from build123d import *

# Parameters (mm, degrees)
ESBO_O1_W                = 20
ESBO_O1_H                = 3.5
RESSALTO_EXTRUS_O1_DEPTH = 22
ESBO_O2_W                = 18
ESBO_O2_H                = 3.80087929
CORTE_EXTRUS_O1_DEPTH    = 20.5
ESBO_O3_W                = 1
ESBO_O3_H                = 20.5
CORTE_EXTRUS_O2_DEPTH    = 1.5
ESBO_O4_W                = 20
ESBO_O4_H                = 1.5
RESSALTO_EXTRUS_O2_DEPTH = 10
ESBO_O5_R                = 1.5
CORTE_EXTRUS_O3_DEPTH    = 7
ESBO_O6_W                = 9
ESBO_O6_H                = 3.518504599
CORTE_EXTRUS_O4_DEPTH    = 2.5


with BuildPart() as part:
    # Esboço1 → Ressalto-extrusão1 (new body)
    with BuildSketch(Plane.XY):
        with Locations((17.16043247, -2.285464773)):
            Rectangle(ESBO_O1_W, ESBO_O1_H)
    extrude(amount=RESSALTO_EXTRUS_O1_DEPTH)

    # Esboço2 → Corte-extrusão1 (cut)
    with BuildSketch(Plane.XY.offset(22)):
        with Locations((17.16043247, -1.135025128)):
            Rectangle(ESBO_O2_W, ESBO_O2_H)
    extrude(amount=-CORTE_EXTRUS_O1_DEPTH, mode=Mode.SUBTRACT)

    # Esboço3 → Corte-extrusão2 (cut)
    with BuildSketch(Plane(origin=(0, -1.535464773, 0), x_dir=(1, 0, 0), z_dir=(0, 1, 0))):
        with Locations((7.66043247, -11.75)):
            Rectangle(ESBO_O3_W, ESBO_O3_H)
        with Locations((26.66043247, -11.75)):
            Rectangle(ESBO_O3_W, ESBO_O3_H)
    extrude(amount=-CORTE_EXTRUS_O2_DEPTH, mode=Mode.SUBTRACT)

    # Esboço4 → Ressalto-extrusão2 (add)
    with BuildSketch(Plane.XZ.offset(4.035464773)):
        with Locations((17.16043247, 0.75)):
            Rectangle(ESBO_O4_W, ESBO_O4_H)
    extrude(amount=RESSALTO_EXTRUS_O2_DEPTH)

    # Esboço5 → Corte-extrusão3 (cut)
    with BuildSketch(Plane.XY.offset(1.5)):
        with Locations((17.16043247, -9.035464773)):
            Circle(ESBO_O5_R)
    extrude(amount=-CORTE_EXTRUS_O3_DEPTH, mode=Mode.SUBTRACT)

    # Esboço6 → Corte-extrusão4 (cut)
    with BuildSketch(Plane(origin=(0, -0.535464773, 0), x_dir=(1, 0, 0), z_dir=(0, 1, 0))):
        with Locations((17.16043247, -0.984028815)):
            Rectangle(ESBO_O6_W, ESBO_O6_H)
    extrude(amount=-CORTE_EXTRUS_O4_DEPTH, mode=Mode.SUBTRACT)


solid = part.part
Geometry: final body of the model. Coordinates: model frame, mm. A direction names the side the tool comes from. Coordinates: 2 decimals unless noted, no trailing zeros. Loops run counter-clockwise (first coordinate to the right, second up) from the corner with the lowest first, then second, coordinate; pieces in that order, holes last. Notation, with made-up numbers: (27, 22) - (47, 22) arc R29 ccw to (47, 43) - close; hole circle Ø7 at (60, 8.5). An arc over 180 degrees is marked (long way). Put each result on its own line as item: value. Start each with the question number.
Q1. Pin query (flat end, axial travel): pin 1 Ø5 at (y, z) = (-6.5, 19) entering from -X; pin 2 Ø1.1 at (x, z) = (8, 15) entering from -Y; pin 3 Ø6 at (x, z) = (22, 13.5) entering from +Y; pin 4 Ø2 at (x, y) = (25, -2) entering from +Z. Return the tip coordinate at first contact, or that it passes through.
Q2. Cut plane B-B, the plane y = -2. Return loops of the section in (x, z).
Q3. Cut plane A-A, the plane z = 18.5. Return loops of the section in (x, y).
Q4. Cut plane D-D, the plane y = -12.25. Return loops of the section in (x, z), and give its area (3 significant figures).
Q5. Cut plane C-C, the plane x = 22.25. Return loops of the section in (y, z).
Q6. Pull-direction query (Y, two-part tool) for faces 6 (the flat face through (8.16, -1, 12)), 7 (the flat face through (8, -1.535, 12)), 8 (the flat face through (27, -0.535, 9)); classes: released by +Y, released by -Y, zero draft, split by the parting line, or undercut.
Q7. Line query: line 1 (Y direction, x = 12.5, z = 12.25); line 2 (Z direction, x = 17.5, y = -12.5). Output: solid intervals per line, ascending.
Q8. Set-up query: faces 1 (the flat face through (27, -1.535, 12)), 2 (the flat face through (27, -1, 22)), 3 (the flat face through (26.16, -1, 12)), 4 (the flat face through (12.66, -2, 1)), 5 (the flat face through (17, -7, 1.5)). Return all of +Z, -Z, +X, -X, +Y, -Y with unobstructed straight access to the full face (end or side cutting, diameter ignored); none if empty.
Filled sheet:
1. pin 1: x = 7.16
1. pin 2: y = -4.04
1. pin 3: y = -3.04
1. pin 4: z = 1.5
2. outline: (7.16, 0) - (12.66, 0) - (12.66, 1.5) - (7.16, 1.5) - close; (21.66, 0) - (27.16, 0) - (27.16, 1.5) - (21.66, 1.5) - close
3. outline: (7.16, -4.04) - (27.16, -4.04) - (27.16, -3.04) - (7.16, -3.04) - close; (7.16, -1.54) - (8.16, -1.54) - (8.16, -0.54) - (7.16, -0.54) - close; (26.16, -1.54) - (27.16, -1.54) - (27.16, -0.54) - (26.16, -0.54) - close
4. outline: (7.16, 0) - (27.16, 0) - (27.16, 1.5) - (7.16, 1.5) - close
4. area: 30.0 mm²
5. outline: (-14.04, 0) - (-0.54, 0) - (-0.54, 1.5) - (-3.04, 1.5) - (-3.04, 22) - (-4.04, 22) - (-4.04, 1.5) - (-14.04, 1.5) - close
6. face 6: zero draft
6. face 7: undercut
6. face 8: released by +Y
7. line 1: -4.04 to -3.04
7. line 2: 0 to 1.5
8. face 1: +Z, +X, -X
8. face 2: +Z, +X, -X, +Y, -Y
8. face 3: +Z, +Y
8. face 4: +Z, -Z, +Y
8. face 5: +Z, +X, -X, -Y
